```python
from build123d import *

# Parameters (mm, degrees)
SKETCH1_R           = 5
BOSS_EXTRUDE1_DEPTH = 15
BOSS_EXTRUDE2_START = 2
SKETCH2_R           = 5
SKETCH2_R_2         = 0.8
BOSS_EXTRUDE2_DEPTH = 2
SKETCH3_R           = 5
BOSS_EXTRUDE3_DEPTH = 3


with BuildPart() as part:
    # Sketch1 → Boss-Extrude1 (new body)
    with BuildSketch(Plane(origin=(0, 0, 0), x_dir=(1, 0, 0), z_dir=(0, 1, 0))):
        with Locations(Location((0, 0, 0), (0, 0, 270))):
            Circle(SKETCH1_R)
        with BuildLine():
            Line((1.5, -2.236067977), (1.5, 2.236067977))
            ThreePointArc((1.5, 2.236067977), (1.795875855, 2.692503442), (2.333333333, 2.608745974))
            ThreePointArc((2.333333333, 2.608745974), (3.5, 0), (2.333333333, -2.608745974))
            ThreePointArc((2.333333333, -2.608745974), (1.795875855, -2.692503442), (1.5, -2.236067977))
        make_face(mode=Mode.SUBTRACT)
        with BuildLine():
            Line((-1.5, -2.236067977), (-1.5, 2.236067977))
            ThreePointArc((-1.5, 2.236067977), (-1.795875855, 2.692503442), (-2.333333333, 2.608745974))
            ThreePointArc((-2.333333333, 2.608745974), (-3.5, 0), (-2.333333333, -2.608745974))
            ThreePointArc((-2.333333333, -2.608745974), (-1.795875855, -2.692503442), (-1.5, -2.236067977))
        make_face(mode=Mode.SUBTRACT)
    extrude(amount=BOSS_EXTRUDE1_DEPTH)

    # Sketch2 → Boss-Extrude2 (add)
    with BuildSketch(Plane.XZ.offset(BOSS_EXTRUDE2_START)):
        with Locations(Location((0, 0, 0), (0, 0, 270))):
            Circle(SKETCH2_R)
        with Locations(Location((-2.5, 0, 0), (0, 0, 270))):
            Circle(SKETCH2_R_2, mode=Mode.SUBTRACT)
        with Locations(Location((2.5, 0, 0), (0, 0, 90))):
            Circle(SKETCH2_R_2, mode=Mode.SUBTRACT)
    extrude(amount=-BOSS_EXTRUDE2_DEPTH)

    # Sketch3 → Boss-Extrude3 (add)
    with BuildSketch(Plane(origin=(0, 15, 0), x_dir=(1, 0, 0), z_dir=(0, 1, 0))):
        with Locations(Location((0, 0, 0), (0, 0, 90))):
            Circle(SKETCH3_R)
    extrude(amount=BOSS_EXTRUDE3_DEPTH)


solid = part.part
```
Work out the finished part from the listing and answer in its coordinate system (mm). A direction names the side the tool comes from. Round coordinates to 2 decimals unless told otherwise and drop trailing zeros. Write each loop counter-clockwise with the first axis right and the second up, starting at its lowest first coordinate (ties: lowest second). Pieces come first, ordered by that corner, then holes. Notation, with made-up numbers: (7, -39) -> (46, -39) arc R21 ccw to (46, -29) -> close; hole circle Ø1 at (85, 46). An arc over 180 degrees is marked (long way). Write each question's results on one line, items separated by ' | '.
Q1. Section B-B, the plane z = 2 is taken. Write down the section's boundary in (x, y).
Data:
outline: (-4.58, -2) -> (4.58, -2) -> (4.58, 18) -> (-4.58, 18) -> close; hole (-2.87, 0) -> (-1.5, 0) -> (-1.5, 15) -> (-2.87, 15) -> close; hole (1.5, 0) -> (2.87, 0) -> (2.87, 15) -> (1.5, 15) -> close
Q2. Section A-A, the plane y = 1.25 is taken. Write down the section's boundary in (x, z).
Data:
outline: circle Ø10 at (0, 0); hole (-2.33, -2.61) arc R0.5 ccw to (-1.5, -2.24) -> (-1.5, 2.24) arc R0.5 ccw to (-2.33, 2.61) arc R3.5 ccw to start; hole (1.5, -2.24) arc R0.5 ccw to (2.33, -2.61) arc R3.5 ccw to (2.33, 2.61) arc R0.5 ccw to (1.5, 2.24) -> close
Q3. Section C-C, the plane z = 0 is taken. Write down the section's boundary in (x, y), then the cut area to 3 significant figures.
Data:
outline: (-5, -2) -> (-3.3, -2) -> (-3.3, 0) -> (-3.5, 0) -> (-3.5, 15) -> (-1.5, 15) -> (-1.5, 0) -> (-1.7, 0) -> (-1.7, -2) -> (1.7, -2) -> (1.7, 0) -> (1.5, 0) -> (1.5, 15) -> (3.5, 15) -> (3.5, 0) -> (3.3, 0) -> (3.3, -2) -> (5, -2) -> (5, 18) -> (-5, 18) -> close | area: 134 mm^2
Q4. Section D-D, the plane z = -1.5 is taken. Write down the section's boundary in (x, y).
Data:
outline: (-4.77, -2) -> (4.77, -2) -> (4.77, 18) -> (-4.77, 18) -> close; hole (-3.16, 0) -> (-1.5, 0) -> (-1.5, 15) -> (-3.16, 15) -> close; hole (1.5, 0) -> (3.16, 0) -> (3.16, 15) -> (1.5, 15) -> close
Q5. Determine the mould class of faces 1 (the cylindrical face through (-3.5, 7.4, 0)), 2 (the flat face through (0, -2, 0)), 3 (the flat face through (1.5, 7, 0)) for opening direction X: released by +X, released by -X, zero draft, split by the parting line, or undercut.
Data:
face 1: undercut | face 2: zero draft | face 3: undercut
Q6. Flat-ended cylindrical pins translate along their axes: P1, Ø1.3, axis at x = -2.5, z = 0, coming from the -Y side; P2, Ø2, axis at x = 3.5, y = 6.5, coming from the +Z side. Find the tip coordinate at first contact, or state that the pin passes through.
Data:
P1: y = 15 | P2: z = 4.33
Q7. Which of the six approach directions +Z, -Z, +X, -X, +Y, -Y give full straight-line access (tool end or side, diameter ignored) to faces 4 (the flat face through (0, 18, 0)), 5 (the cylindrical face through (3.28, -1.01, -0.17)), 6 (the flat face through (-2, 0, -1))?
Data:
face 4: +Z, -Z, +X, -X, +Y | face 5: -Y | face 6: none
Q8. Straight lines are drawn through the part: line 1 along X through (y, z) = (12.75, 0); line 2 along X through (y, z) = (-1.45, 0); line 3 along Y through (x, z) = (2.25, 2.25). For each, find the intervals that lie inside material, in ascending order. Write a range as [from, to].
Data:
line 1: [-5, -3.5], [-1.5, 1.5], [3.5, 5] | line 2: [-5, -3.3], [-1.7, 1.7], [3.3, 5] | line 3: [-2, 0], [15, 18]
